from build123d import *

# Parameters (mm, degrees)
SKETCH010_AS_DRAWN_R                      = 3
EXTRUDE009_DEPTH                          = 40
EXTRUDE009_ONTO_SKETCH010_PLACEMENT_ANGLE = 9
EXTRUDE001_DEPTH                          = 5
EXTRUDE001_PLACEMENT_ANGLE                = 45


with BuildPart() as extrude009:
    # Sketch010 as drawn → Extrude009 (new)
    with BuildSketch(Plane.XY):
        Circle(SKETCH010_AS_DRAWN_R)
    extrude(amount=-EXTRUDE009_DEPTH)


with BuildPart() as extrude009_1:
    # Extrude009 onto Sketch010 placement: moved
    add(extrude009.part.moved(Location((-32, -32, 30))).rotate(Axis((-32, -32, 30), (0, 0, -1)), EXTRUDE009_ONTO_SKETCH010_PLACEMENT_ANGLE))


with BuildPart() as cut003:
    # Sketch001 (on Face7 of Extrude) → Extrude001 (new body)
    with BuildSketch(Plane.XY.offset(17)):
        with BuildLine():
            Line((25, 0), (25, 70))
            Line((25, 70), (-25, 70))
            Line((-25, 70), (-25, 0))
            ThreePointArc((25, 0), (0, 25), (-25, 0))
        make_face()
    extrude(amount=-EXTRUDE001_DEPTH)


with BuildPart() as cut003_1:
    # Extrude001 placement: moved
    add(cut003.part.rotate(Axis((0, 0, 0), (0, 0, -1)), EXTRUDE001_PLACEMENT_ANGLE))

    # Cut003: cut Extrude009
    add(extrude009_1.part, mode=Mode.SUBTRACT)


solid = cut003_1.part
Can you work these out from the model? Positions are in its coordinate system, mm. Coordinates: 2 decimals unless noted, no trailing zeros. Loops run counter-clockwise (first coordinate to the right, second up) from the corner with the lowest first, then second, coordinate; pieces in that order, holes last. Notation, with made-up numbers: M 39,-34 L 71,-34 A18 ccw 71,-1 Z; hole C 14,88.25 d7. An arc over 180 degrees is marked long. Return JSON: item names as keys, results as strings. Group by question number.
Item 1: Imagine slicing it at D-D (x = 47). Please give me the cut outline in (y, z), and give its area (3 significant figures).
Item 2: I'm going to push flat-ended pins straight in: pin 1 Ø1 at (y, z) = (29, 16) entering from -X; pin 2 Ø2 at (x, z) = (27.5, 15) entering from -Y; pin 3 Ø1.5 at (x, z) = (7, 14.5) entering from +Y. Where does each tip first touch, or does it pass through?
Item 3: Imagine slicing it at B-B (y = 21). Please give me the cut outline in (x, z), and give its area (3 significant figures).
Item 4: Imagine slicing it at A-A (x = 19). Please give me the cut outline in (y, z).
Item 5: If I drill on L1, parallel to Y at x = 19.5, z = 12.95; L2, parallel to Y at x = -13.5, z = 13.05; L3, parallel to Y at x = 33.5, z = 16.6, over which ranges is the centre line in solid material (lowest first)? Write a range as from..to.
Item 6: Imagine slicing it at C-C (z = 13.9). Please give me the cut outline in (x, y).
Verdict:
{
 "1": {"outline": "M 11.64,12 L 51.99,12 L 51.99,17 L 11.64,17 Z", "area": "202 mm^2"},
 "2": {"pin 1": "stops at x = -6.86", "pin 2": "stops at y = -8.86", "pin 3": "stops at y = 43.11"},
 "3": {"outline": "M -14.36,12 L -13.56,12 L -13.56,17 L -14.36,17 Z; M 13.56,12 L 56.36,12 L 56.36,17 L 13.56,17 Z", "area": "218 mm^2"},
 "4": {"outline": "M -16.36,12 L -16.25,12 L -16.25,17 L -16.36,17 Z; M 16.25,12 L 54.36,12 L 54.36,17 L 16.25,17 Z"},
 "5": {"L1": "y = -15.86..-15.64, 15.64..54.86", "L2": "y = 21.04..21.86", "L3": "y = -1.86..65.49"},
 "6": {"outline": "M -17.68,17.68 A25 cw 17.68,-17.68 L 67.18,31.82 L 31.82,67.18 Z"}
}
